```python
from build123d import *

# Parameters (mm, degrees)
SKETCH1_W           = 1422.4
SKETCH1_H           = 762
BOSS_EXTRUDE1_DEPTH = 76.2
SKETCH3_W           = 101.6
SKETCH3_H           = 101.6
CUT_EXTRUDE1_DEPTH  = 38.1


with BuildPart() as part:
    # Sketch1 → Boss-Extrude1 (new body)
    with BuildSketch(Plane(origin=(0, 0, 0), x_dir=(1, 0, 0), z_dir=(0, 1, 0))):
        with Locations((711.2, 381)):
            Rectangle(SKETCH1_W, SKETCH1_H)
    extrude(amount=BOSS_EXTRUDE1_DEPTH)

    # Sketch3 → Cut-Extrude1 (cut)
    with BuildSketch(Plane.XZ):
        with Locations((152.4, -101.6)):
            Rectangle(SKETCH3_W, SKETCH3_H)
        with Locations((152.4, -660.4)):
            Rectangle(SKETCH3_W, SKETCH3_H)
        with Locations((1270, -101.6)):
            Rectangle(SKETCH3_W, SKETCH3_H)
        with Locations((1270, -660.4)):
            Rectangle(SKETCH3_W, SKETCH3_H)
    extrude(amount=-CUT_EXTRUDE1_DEPTH, mode=Mode.SUBTRACT)


solid = part.part
```
Geometry check sheet. Reference: the model listing, model coordinates, mm. A direction names the side the tool comes from. Give positions to 0.01 mm unless a question says otherwise; leave off trailing zeros. Write each loop counter-clockwise with the first axis right and the second up, starting at its lowest first coordinate (ties: lowest second). Pieces come first, ordered by that corner, then holes.
1) Section check C-C, the plane x = 186.5. Record the boundary of the cut face in (y, z).
2) Material ranges on L1, parallel to X at y = 24.5, z = -56.5; L2, parallel to Y at x = 119, z = -688.5, recorded low to high.
3) Release check for a two-part mould opening along Z. For faces 3 (the flat face through (701, 0, -386)), 4 (the flat face through (1269, 19, -152.4)), 5 (the flat face through (701, 38, 0)) record: pulls with the +Z half, pulls with the -Z half, needs draft (parallel to the pull), parting line crosses it, or undercut.
4) Section check B-B, the plane y = 18. Record the boundary of the cut face in (x, z), and give its area (3 significant figures).
5) Access from +Z, -Z, +X, -X, +Y, -Y to the whole of each face (thin tool, end or side, straight path). Record for faces 1 (the flat face through (1269, 38.1, -101)), 2 (the flat face through (1422.4, 38, -376)).
6) Section check A-A, the plane z = -119. Record the boundary of the cut face in (x, y).
Computed:
1. outline: (0, -762) - (76.2, -762) - (76.2, 0) - (0, 0) - (0, -50.8) - (38.1, -50.8) - (38.1, -152.4) - (0, -152.4) - (0, -609.6) - (38.1, -609.6) - (38.1, -711.2) - (0, -711.2) - close
2. L1: x = 0 to 101.6, 203.2 to 1219.2, 1320.8 to 1422.4
2. L2: y = 38.1 to 76.2
3. face 3: needs draft
3. face 4: undercut
3. face 5: pulls with the +Z half
4. outline: (0, -762) - (1422.4, -762) - (1422.4, 0) - (0, 0) - close; hole (101.6, -711.2) - (203.2, -711.2) - (203.2, -609.6) - (101.6, -609.6) - close; hole (101.6, -152.4) - (203.2, -152.4) - (203.2, -50.8) - (101.6, -50.8) - close; hole (1219.2, -711.2) - (1320.8, -711.2) - (1320.8, -609.6) - (1219.2, -609.6) - close; hole (1219.2, -152.4) - (1320.8, -152.4) - (1320.8, -50.8) - (1219.2, -50.8) - close
4. area: 1,040,000 mm2
5. face 1: -Y
5. face 2: +Z, -Z, +X, +Y, -Y
6. outline: (0, 0) - (101.6, 0) - (101.6, 38.1) - (203.2, 38.1) - (203.2, 0) - (1219.2, 0) - (1219.2, 38.1) - (1320.8, 38.1) - (1320.8, 0) - (1422.4, 0) - (1422.4, 76.2) - (0, 76.2) - close
